from build123d import *

# Parameters (mm, degrees)
SKETCH2_W          = 50
SKETCH2_H          = 92.5
BASE_FLANGE1_DEPTH = 2
SKETCH1_R          = 2.5
SKETCH1_R_2        = 5
SKETCH1_R_3        = 17.1
CUT_EXTRUDE1_DEPTH = 10


# Sheet-metal steps are written as plain solids
with BuildPart() as part:
    # Sketch2 → Base-Flange1 (new body)
    with BuildSketch(Plane(origin=(0, 0, 0), x_dir=(1, 0, 0), z_dir=(0, 1, 0))):
        with Locations((-2.5, -1.25)):
            Rectangle(SKETCH2_W, SKETCH2_H)
    extrude(amount=-BASE_FLANGE1_DEPTH)

    # Sketch1 → Cut-Extrude1 (cut)
    with BuildSketch(Plane(origin=(0, 0, 0), x_dir=(1, 0, 0), z_dir=(0, 1, 0))):
        with Locations(Location((-16.25, 11.74, 0), (0, 0, 270))):
            Circle(SKETCH1_R)
        with Locations(Location((11.25, 11.74, 0), (0, 0, 270))):
            Circle(SKETCH1_R)
        with Locations(Location((11.25, 32.5, 0), (0, 0, 270))):
            Circle(SKETCH1_R)
        with Locations(Location((-19.25, -38.5, 0), (0, 0, 270))):
            Circle(SKETCH1_R_2)
        with Locations(Location((14.25, -38.5, 0), (0, 0, 270))):
            Circle(SKETCH1_R_2)
        with Locations(Location((14.25, -6, 0), (0, 0, 270))):
            Circle(SKETCH1_R_2)
        with Locations(Location((-19.25, -6, 0), (0, 0, 270))):
            Circle(SKETCH1_R_2)
        with Locations(Location((-16.25, 32.5, 0), (0, 0, 270))):
            Circle(SKETCH1_R)
        with Locations(Location((-2.5, -22.25, 0), (0, 0, 270))):
            Circle(SKETCH1_R_3)
    extrude(amount=-CUT_EXTRUDE1_DEPTH, mode=Mode.SUBTRACT)


solid = part.part
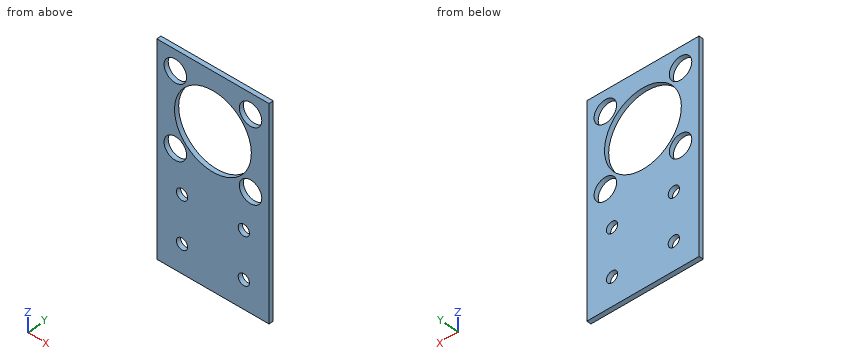
Geometry check sheet. Reference: the model listing, model coordinates, mm. Coordinates: 2 decimals unless noted, no trailing zeros. Order: outer loops, then holes, each group sorted by start corner. A loop starts at its lowest first (then second) coordinate and runs counter-clockwise, first axis right, second up. Notation, with made-up numbers: M -1,79.5 L 28,79.5 A17 cw 28,110.5 Z; hole C 7.25,75 d5. An arc over 180 degrees is marked long. Use CSV: the item, a comma, the result in double quotes.
Item 1: Cross-section at D-D on x = -22.5. Record the cut outline in (y, z), then the cut area to 3 significant figures.
Returned:
outline,"M -2,-45 L 0,-45 L 0,2.2 L -2,2.2 Z; M -2,9.8 L 0,9.8 L 0,34.7 L -2,34.7 Z; M -2,42.3 L 0,42.3 L 0,47.5 L -2,47.5 Z"
area,"155 mm2"
Item 2: Cross-section at B-B on z = -31. Record the cut outline in (x, y).
Returned:
outline,"M -27.5,-2 L -18.25,-2 L -18.25,0 L -27.5,0 Z; M -14.25,-2 L 9.25,-2 L 9.25,0 L -14.25,0 Z; M 13.25,-2 L 22.5,-2 L 22.5,0 L 13.25,0 Z"
Item 3: Gauge pin test, flat end, axial feed: pin 1 Ø10 at (x, z) = (11.5, 32.5) entering from +Y. Record the tip position at first contact, or that the pin passes through.
Returned:
pin 1,"stops at y = 0"
Item 4: Thickness scan on line 1 along X through (y, z) = (-1.65, -11.5); line 2 along Z through (x, y) = (-16, -1.5); line 3 along X through (y, z) = (-1.2, 38). Record the ranges inside material, lowest first.
Returned:
line 1,"x = -27.5 to -18.74, -13.76 to 8.76, 13.74 to 22.5"
line 2,"z = -45 to -34.99, -30.01 to -14.23, -9.25 to 2.2, 9.8 to 11.75, 32.75 to 34.7, 42.3 to 47.5"
line 3,"x = -27.5 to -24.22, -14.28 to -9.16, 4.16 to 9.28, 19.22 to 22.5"
Item 5: Cross-section at A-A on x = -2.5. Record the cut outline in (y, z), then the cut area to 3 significant figures.
Returned:
outline,"M -2,-45 L 0,-45 L 0,5.15 L -2,5.15 Z; M -2,39.35 L 0,39.35 L 0,47.5 L -2,47.5 Z"
area,"117 mm2"
Item 6: Cross-section at C-C on z = 22.25. Record the cut outline in (x, y).
Returned:
outline,"M -27.5,-2 L -19.6,-2 L -19.6,0 L -27.5,0 Z; M 14.6,-2 L 22.5,-2 L 22.5,0 L 14.6,0 Z"
